from build123d import *

# Parameters (mm, degrees)
SCHIZZO1_R                   = 1.6
ESTRUSIONE_ESTRUSIONE1_DEPTH = 45
SCHIZZO2_R                   = 1.6
ESTRUSIONE_ESTRUSIONE2_DEPTH = 5
ESTRUSIONE_ESTRUSIONE2_DRAFT = -4.6
SCHIZZO3_R                   = 2.002290448
ESTRUSIONE_ESTRUSIONE3_DEPTH = 3


with BuildPart() as part:
    # Schizzo1 → Estrusione-Estrusione1 (new body)
    with BuildSketch(Plane(origin=(0, 0, 0), x_dir=(0, 1, 0), z_dir=(0, 0, 1))):
        with Locations(Location((0, 0, 0), (0, 0, 90))):
            Circle(SCHIZZO1_R)
    extrude(amount=ESTRUSIONE_ESTRUSIONE1_DEPTH)


with BuildPart() as estrusione_estrusione2_tool:
    # Schizzo2 → Estrusione-Estrusione2 (with draft: the straight prism first)
    with BuildSketch(Plane.XY.offset(45)):
        with Locations(Location((0, 0, 0), (0, 0, 180))):
            Circle(SCHIZZO2_R)
    extrude(amount=ESTRUSIONE_ESTRUSIONE2_DEPTH)
    # Estrusione-Estrusione2: the draft: its side faces are tilted about the plane it starts from
    estrusione_estrusione2_sides = [estrusione_estrusione2_tool.faces().sort_by_distance(p)[0] for p in [
        (1.6, 0, 47.5),
    ]]
    draft(estrusione_estrusione2_sides, Plane.XY.offset(45), ESTRUSIONE_ESTRUSIONE2_DRAFT)


with BuildPart() as part_1:
    add(part.part)

    # Estrusione-Estrusione2: add estrusione_estrusione2_tool
    add(estrusione_estrusione2_tool.part)

    # Schizzo3 → Estrusione-Estrusione3 (add)
    with BuildSketch(Plane.XY.offset(50)):
        Circle(SCHIZZO3_R)
    extrude(amount=ESTRUSIONE_ESTRUSIONE3_DEPTH)


solid = part_1.part
Check sheet for the modelled part. Datum: model origin and axes. Units: mm. A direction names the side the tool comes from. Give positions to 0.01 mm unless a question says otherwise; leave off trailing zeros. Write each loop counter-clockwise with the first axis right and the second up, starting at its lowest first coordinate (ties: lowest second). Pieces come first, ordered by that corner, then holes. Notation, with made-up numbers: (65.25, -22.5) -> (89.25, -22.5) arc R17 cw to (89.25, 5.5) -> close; hole circle Ø3 at (63, 80.25). An arc over 180 degrees is marked (long way). One line per item, written item: value. Start each with the question number.
Item 1: Tool access check on faces 1 (the cylindrical face through (1.27, 0.97, 22.18)), 2 (the flat face through (0, 0, 0)). Record the directions out of +Z, -Z, +X, -X, +Y, -Y that give a thin tool (end or side, any length) a straight path to the whole face; none if there is none.
Item 2: Material ranges on probe 1 along X at (y, z) = (0.05, 42); probe 2 along Y at (x, z) = (1.2, 7), recorded low to high. Write a range as from..to.
Item 3: Gauge pin test, flat ends, axial feed: pin 1 (2 mm diameter, centred on y = 0.5, z = 42, fed in from -X); pin 2 (1.5 mm diameter, centred on x = 0.5, z = 16.5, fed in from -Y); pin 3 (1.5 mm diameter, centred on x = -0.5, z = 43.5, fed in from +Y). Record the tip position at first contact, or that the pin passes through.
Item 4: Section check A-A on x = 0. Record the cut outline in (y, z).
Item 5: Section check C-C on z = 38. Record the cut outline in (x, y).
Results list:
1. face 1: -Z
1. face 2: -Z, +X, -X, +Y, -Y
2. probe 1: -1.6..1.6
2. probe 2: -1.06..1.06
3. pin 1: x = -1.6
3. pin 2: y = -1.6
3. pin 3: y = 1.6
4. outline: (-2, 50) -> (-1.6, 45) -> (-1.6, 0) -> (1.6, 0) -> (1.6, 45) -> (2, 50) -> (2, 53) -> (-2, 53) -> close
5. outline: circle Ø3.2 at (0, 0)
